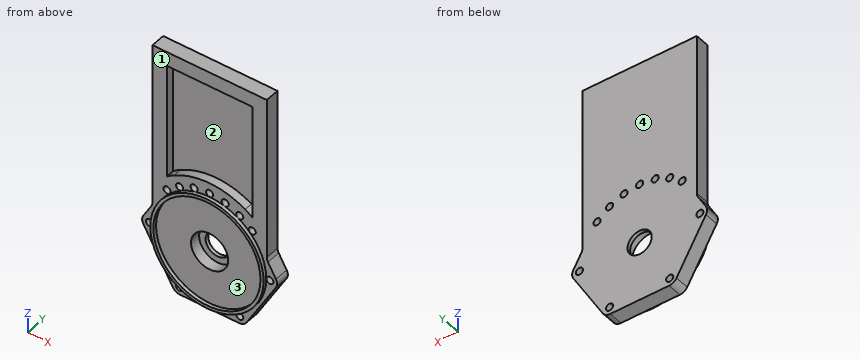
Autodesk Inventor part; units mm, degrees
ref_plane "YZ Plane" through (0, 0, 0) normal (1, 0, 0) x (0, 1, 0)
ref_plane "XZ Plane" through (0, 0, 0) normal (0, 1, 0) x (-1, 0, 0)
ref_plane "XY Plane" through (0, 0, 0) normal (0, 0, 1) x (1, 0, 0)
sketch "Sketch1" plane through (0, 0, 0) normal (0, 1, 0) x (-1, 0, 0)
  line L0 (83.678612, 197.794487) -> (-76.321388, 197.794487)
  line L1 (-76.321388, 197.794487) -> (-76.321388, -52.205513)
  line L2 (-76.321388, -52.205513) -> (83.678612, -52.205513)
  line L3 (83.678612, -52.205513) -> (83.678612, 197.794487)
  circle A0 centre (3.678612, -62.205513) radius 80
  line L4 (83.678612, -52.205513) -> (83.678612, -62.205513)
  line L5 (-76.321388, -52.205513) -> (-76.321388, -62.205513)
  circle A1 centre (3.678612, -62.205513) radius 26
  circle A2 centre (3.678612, -62.205513) radius 40
  point P0 (0, 0)
  point P1 (59.392898, -23.634084)
  point P2 (-75.693927, -52.205513)
  point P3 (83.051152, -52.205513)
  dimension "d0" = 250
  dimension "d1" = 160
  dimension "d2" = 160
  dimension "d3" = 10
  dimension "d4" = 52
  dimension "d5" = 80
extrude "Extrusion1" add sketch "Sketch1" along normal blind 20 contours L3 L2 A0 L1 L0 | L4 A0 L2 | L2 A0 L5 | A0 L2 A2 | L2 A2 A0 | A2 L2 A1 | L2 A1 A2
sketch "Sketch2" plane through (0, 20, 0) normal (0, 1, 0) x (1, 0, 0)
  circle A0 centre (-3.678612, 62.205513) radius 26
  circle A1 centre (-3.678612, 62.205513) radius 26
  circle A2 centre (-3.678612, 62.205513) radius 17
  point P0 (0, 0)
  dimension "d8" = 34
extrude "Extrusion2" add sketch "Sketch2" against normal blind 5
sketch "Sketch3" plane through (0, 0, 0) normal (0, -1, 0) x (1, 0, 0)
  circle A0 centre (-3.678612, -62.205513) radius 75
  circle A1 centre (-3.678612, -62.205513) radius 75
  line L0 (92.607102, -62.205513) -> (44.464245, -145.591387)
  line L1 (44.464245, -145.591387) -> (-51.821469, -145.591387)
  line L2 (-51.821469, -145.591387) -> (-99.964327, -62.205513)
  line L3 (-99.964327, -62.205513) -> (-51.821469, 21.180362)
  line L4 (-51.821469, 21.180362) -> (44.464245, 21.180362)
  line L5 (44.464245, 21.180362) -> (92.607102, -62.205513)
  line L6 (80.607102, -62.205513) -> (38.464245, -135.199083)
  line L7 (38.464245, -135.199083) -> (-45.821469, -135.199083)
  line L8 (-45.821469, -135.199083) -> (-87.964327, -62.205513)
  line L9 (-87.964327, -62.205513) -> (-45.821469, 10.788057)
  line L10 (-45.821469, 10.788057) -> (38.464245, 10.788057)
  line L11 (38.464245, 10.788057) -> (80.607102, -62.205513)
  circle A2 centre (80.607102, -62.205513) radius 5
  circle A3 centre (38.464245, 10.788057) radius 5
  circle A4 centre (-45.821469, 10.788057) radius 5
  circle A5 centre (-87.964327, -62.205513) radius 5
  circle A6 centre (-45.821469, -135.199083) radius 5
  circle A7 centre (38.464245, -135.199083) radius 5
  circle A8 centre (-3.678612, -62.205513) radius 26
  circle A9 centre (-3.678612, -62.205513) radius 0.853538
  point P0 (0, 0)
  point P1 (-59.392898, -100.776941)
  point P2 (-3.678612, -62.205513)
  dimension "d13" = 360
sketch "Sketch4" plane through (0, 0, 0) normal (0, -1, 0) x (1, 0, 0)
  circle A0 centre (-45.821469, -135.199083) radius 5
  line L0 (-45.821469, -135.199083) -> (-87.964327, -62.205513)
  line L1 (-51.821469, -145.591387) -> (-99.964327, -62.205513)
  circle A1 centre (-87.964327, -62.205513) radius 5
  circle A2 centre (-45.821469, 10.788057) radius 5
  line L2 (-87.964327, -62.205513) -> (-45.821469, 10.788057)
  line L3 (-99.964327, -62.205513) -> (-51.821469, 21.180362)
  line L4 (38.464245, -135.199083) -> (-45.821469, -135.199083)
  circle A3 centre (38.464245, -135.199083) radius 5
  line L5 (44.464245, -145.591387) -> (-51.821469, -145.591387)
  line L6 (80.607102, -62.205513) -> (38.464245, -135.199083)
  line L7 (92.607102, -62.205513) -> (44.464245, -145.591387)
  circle A4 centre (-3.678612, -62.205513) radius 75
  circle A5 centre (-3.678612, -62.205513) radius 75
  line L8 (-45.821469, 10.788057) -> (38.464245, 10.788057)
  line L9 (-51.821469, 21.180362) -> (44.464245, 21.180362)
  circle A6 centre (80.607102, -62.205513) radius 5
  circle A7 centre (38.464245, 10.788057) radius 5
  line L10 (38.464245, 10.788057) -> (80.607102, -62.205513)
  line L11 (44.464245, 21.180362) -> (92.607102, -62.205513)
  circle A8 centre (-3.678612, -62.205513) radius 26
  circle A9 centre (-3.678612, -62.205513) radius 17
  circle A10 centre (-3.678612, -62.205513) radius 2.321388
  point P0 (0, 0)
  point P1 (0, 0)
  point P2 (-59.392898, -100.776941)
  dimension "d18" = 360
extrude "Extrusion3" cut sketch "Sketch3" against normal blind 22 contours A2 L6 L11 | L11 L6 A2 | A3 L10 L11 | L11 L10 A3 | A7 L7 L6 | L6 L7 A7 | A4 L9 L10 | L10 L9 A4 | A6 L8 L7 | L7 L8 A6 | A5 L8 L9 | L9 L8 A5
extrude "Extrusion4" add sketch "Sketch4" against normal blind 20 contours A0 L0 A4 L4 | A4 L6 A3 L4 | L0 A1 L2 A4 | A4 L10 A6 L6 | L2 A2 L8 A4 | L8 A7 L10 A4 | L1 L3 L9 L11 L7 L5
sketch "Sketch5" plane through (0, 0, 0) normal (0, -1, 0) x (1, 0, 0)
  circle A0 centre (-3.678612, -62.205513) radius 17
  circle A1 centre (-3.678612, -62.205513) radius 79.285714
  circle A2 centre (80.607102, -62.205513) radius 5
  circle A3 centre (-3.678612, -62.205513) radius 75
  point P0 (0, 0)
  dimension "d21" = 150
extrude "Extrusion5" add sketch "Sketch5" along normal blind 5 contours A1
fillet "Fillet1" radius 12 6 edges at (-83.6786, 10, -33.9978) (-99.9643, 10, -62.2055) (-51.8215, 10, -145.5914) (44.4642, 10, -145.5914) (92.6071, 10, -62.2055) (76.3214, 10, -33.9978)
sketch "Sketch6" plane through (0, 0, 0) normal (0, -1, 0) x (1, 0, 0)
  arc A0 (89.143, -68.205513) -> (89.143, -56.205513) centre (78.750696, -62.205513) ccw
  line L0 (89.143, -56.205513) -> (77.929083, -36.782438)
  arc A1 (76.321388, -30.782438) -> (77.929083, -36.782438) centre (88.321388, -30.782438) ccw
  line L1 (76.321388, 197.794487) -> (76.321388, -30.782438)
  line L2 (-83.678612, 197.794487) -> (76.321388, 197.794487)
  line L3 (-83.678612, -30.782438) -> (-83.678612, 197.794487)
  arc A2 (-85.286307, -36.782438) -> (-83.678612, -30.782438) centre (-95.678612, -30.782438) ccw
  line L4 (-85.286307, -36.782438) -> (-96.500225, -56.205513)
  arc A3 (-96.500225, -56.205513) -> (-96.500225, -68.205513) centre (-86.10792, -62.205513) ccw
  line L5 (-96.500225, -68.205513) -> (-55.285571, -139.591387)
  arc A4 (-55.285571, -139.591387) -> (-44.893266, -145.591387) centre (-44.893266, -133.591387) ccw
  line L6 (-44.893266, -145.591387) -> (37.536042, -145.591387)
  arc A5 (37.536042, -145.591387) -> (47.928346, -139.591387) centre (37.536042, -133.591387) ccw
  line L7 (47.928346, -139.591387) -> (89.143, -68.205513)
  circle A6 centre (-87.964327, -62.205513) radius 5
  arc A7 (-43.321469, 6.45793) -> (-82.964327, -62.205513) centre (-3.678612, -62.205513) ccw
  circle A8 centre (-45.821469, 10.788057) radius 5
  arc A9 (35.964245, 6.45793) -> (-43.321469, 6.45793) centre (-3.678612, -62.205513) ccw
  circle A10 centre (38.464245, 10.788057) radius 5
  arc A11 (75.607102, -62.205513) -> (35.964245, 6.45793) centre (-3.678612, -62.205513) ccw
  circle A12 centre (80.607102, -62.205513) radius 5
  arc A13 (35.964245, -130.868956) -> (75.607102, -62.205513) centre (-3.678612, -62.205513) ccw
  circle A14 centre (38.464245, -135.199083) radius 5
  arc A15 (-43.321469, -130.868956) -> (35.964245, -130.868956) centre (-3.678612, -62.205513) ccw
  circle A16 centre (-45.821469, -135.199083) radius 5
  arc A17 (-82.964327, -62.205513) -> (-43.321469, -130.868956) centre (-3.678612, -62.205513) ccw
  arc A18 (56.321388, -30.782438) -> (60.608575, -46.782438) centre (88.321388, -30.782438) ccw
  line L8 (60.608575, -46.782438) -> (69.513091, -62.205513)
  line L9 (69.513091, -62.205513) -> (32.917239, -125.591387)
  line L10 (32.917239, -125.591387) -> (-40.274464, -125.591387)
  line L11 (-40.274464, -125.591387) -> (-76.870316, -62.205513)
  line L12 (-76.870316, -62.205513) -> (-67.965799, -46.782438)
  arc A19 (-67.965799, -46.782438) -> (-63.678612, -30.782438) centre (-95.678612, -30.782438) ccw
  line L13 (-63.678612, -30.782438) -> (-63.678612, 177.794487)
  line L14 (-63.678612, 177.794487) -> (56.321388, 177.794487)
  line L15 (56.321388, 177.794487) -> (56.321388, -30.782438)
  arc A20 (-53.321469, 23.778438) -> (-102.964327, -62.205513) centre (-3.678612, -62.205513) ccw
  arc A21 (-102.964327, -62.205513) -> (-53.321469, -148.189464) centre (-3.678612, -62.205513) ccw
  arc A22 (-53.321469, -148.189464) -> (45.964245, -148.189464) centre (-3.678612, -62.205513) ccw
  arc A23 (45.964245, -148.189464) -> (95.607102, -62.205513) centre (-3.678612, -62.205513) ccw
  arc A24 (95.607102, -62.205513) -> (45.964245, 23.778438) centre (-3.678612, -62.205513) ccw
  arc A25 (45.964245, 23.778438) -> (-53.321469, 23.778438) centre (-3.678612, -62.205513) ccw
  point P0 (0, 0)
  point P1 (-63.678612, 16.899816)
  point P2 (56.321388, 16.899816)
  dimension "d25" = 20
  dimension "d26" = 20
sketch "Sketch6 outline for Extrusion6" plane through (0, 0, 0) normal (0, -1, 0) x (1, 0, 0)
  line L0 (56.321388, 177.794487) -> (-63.678612, 177.794487)
  line L1 (56.321388, 16.899816) -> (56.321388, 177.794487)
  arc A0 (45.964245, 23.778438) -> (56.321388, 16.899816) centre (-3.678612, -62.205513) cw
  arc A1 (-53.321469, 23.778438) -> (45.964245, 23.778438) centre (-3.678612, -62.205513) cw
  arc A2 (-63.678612, 16.899816) -> (-53.321469, 23.778438) centre (-3.678612, -62.205513) cw
  line L2 (-63.678612, 177.794487) -> (-63.678612, 16.899816)
extrude "Extrusion6" cut sketch "Sketch6 outline for Extrusion6" against normal blind 12
sketch "Sketch7" plane through (0, 0, 0) normal (0, -1, 0) x (1, 0, 0)
  circle A0 centre (-3.678612, 22.080487) radius 5
  circle A1 centre (-3.678612, -62.205513) radius 17
  circle A2 centre (-25.493434, 19.208511) radius 5
  circle A3 centre (-45.821612, 10.788304) radius 5
  circle A4 centre (-63.277814, -2.606311) radius 5
  circle A5 centre (-76.672429, -20.062513) radius 5
  circle A6 centre (-85.092637, -40.390691) radius 5
  circle A7 centre (-87.964612, -62.205513) radius 5
  circle A8 centre (-85.092637, -84.020335) radius 5
  circle A9 centre (-76.672429, -104.348513) radius 5
  circle A10 centre (-63.277814, -121.804715) radius 5
  circle A11 centre (-45.821612, -135.19933) radius 5
  circle A12 centre (-25.493434, -143.619537) radius 5
  circle A13 centre (-3.678612, -146.491513) radius 5
  circle A14 centre (18.13621, -143.619537) radius 5
  circle A15 centre (38.464388, -135.19933) radius 5
  circle A16 centre (55.92059, -121.804715) radius 5
  circle A17 centre (69.315205, -104.348513) radius 5
  circle A18 centre (77.735412, -84.020335) radius 5
  circle A19 centre (80.607388, -62.205513) radius 5
  circle A20 centre (77.735412, -40.390691) radius 5
  circle A21 centre (69.315205, -20.062513) radius 5
  circle A22 centre (55.92059, -2.606311) radius 5
  circle A23 centre (38.464388, 10.788304) radius 5
  circle A24 centre (18.13621, 19.208511) radius 5
  point P0 (0, 0)
  dimension "d29" = 84.286
  dimension "d30" = 10
  dimension "d33" = 360
extrude "Extrusion7" cut sketch "Sketch7" against normal blind 39 contours A0 | A2 | A4 | A5 | A21 | A22 | A24
sketch "Sketch8" plane through (0, 20, 0) normal (0, 1, 0) x (1, 0, 0)
  circle A0 centre (69.315205, 20.062513) radius 5
  circle A1 centre (-76.672429, 20.062513) radius 5
  point P0 (0, 0)
extrude "Extrusion8" add sketch "Sketch8" against normal blind 20
properties part number "ZadKriska"
Here's how the part is built. I have some questions about the finished solid (model axes, mm). Face numbers are marked on the shaded views. A direction names the side the tool comes from. Round coordinates to 2 decimals unless told otherwise and drop trailing zeros. Order: outer loops, then holes, each group sorted by start corner. A loop starts at its lowest first (then second) coordinate and runs counter-clockwise, first axis right, second up. Notation, with made-up numbers: M 32,22 L 63,22 A33 cw 63,60 Z; hole C -29,48 d1. An arc over 180 degrees is marked long. Return JSON: item names as keys, results as strings. Group by question number.
1. If we section it at B-B on z = -50: List the corners of the cut face in (x, y) for me, then the cut area to 3 significant figures.
2. If we section it at A-A on z = 153: List the corners of the cut face in (x, y) for me.
3. On a 3-axis mill with a long thin cutter (end or side, diameter ignored), from which of +Z, -Z, +X, -X, +Y, -Y can I reach the whole of each face in a straight line? I mean the marked faces 3 and 4. Say none if no direction works.
4. Please list where these lines run through material, in increasing order: probe 1 along Z at (x, y) = (-4.5, 17.5); probe 2 along Z at (x, y) = (-4.5, -3.25); probe 3 along Z at (x, y) = (-50, 2).
5. If we section it at C-C on y = 4.75: State how many separate pieces and enclosed holes the cut face has, then the cut area to 3 significant figures.
6. If we section it at D-D on x = 28: List the corners of the cut face in (y, z) for me.
7. I'm going to push flat-ended pins straight in: pin 1 Ø8 at (x, z) = (80.61, -62.21) entering from -Y; pin 2 Ø11.5 at (x, z) = (-87.96, -62.21) entering from +Y; pin 3 Ø5 at (y, z) = (-0.5, 115.5) entering from +X; pin 4 Ø3 at (x, z) = (18.5, 63.5) entering from -Y. Where does each tip first touch, or does it pass through?
8. If we mould it in two halves opening along X, with no side actions, what happens to the marked faces 1 and 2? For each: pulls with the +X half, pulls with the -X half, needs draft (parallel to the pull), parting line crosses it, or undercut.
Reply:
{
 "1": {"outline": "M -92.92,0 L -82.02,0 L -82.02,-5 L -77.68,-5 L -77.68,0 L -26.64,0 L -26.64,15 L -15.51,15 L -15.51,20 L -92.92,20 Z; M 8.15,15 L 19.28,15 L 19.28,0 L 70.32,0 L 70.32,-5 L 74.66,-5 L 74.66,0 L 85.56,0 L 85.56,20 L 8.15,20 Z", "area": "2,810 mm^2"},
 "2": {"outline": "M -83.68,0 L -63.68,0 L -63.68,12 L 56.32,12 L 56.32,0 L 76.32,0 L 76.32,20 L -83.68,20 Z"},
 "3": {"face 3": "-Y", "face 4": "+Z, -Z, +X, -X, +Y"},
 "4": {"probe 1": "-145.59 to -79.19, -45.23 to 17.15, 27.01 to 197.79", "probe 2": "-141.49 to -137.2, 12.79 to 17.08", "probe 3": "-144.45 to -137.94, -132.45 to 8.04, 13.53 to 25.61, 177.79 to 197.79"},
 "5": {"separate pieces": "1", "enclosed holes": "13", "area": "33,400 mm^2"},
 "6": {"outline": "M -5,-134.89 L 0,-134.89 L 0,-145.59 L 20,-145.59 L 20,197.79 L 0,197.79 L 0,177.79 L 12,177.79 L 12,31.89 L 0,31.89 L 0,10.48 L -5,10.48 L -5,5.78 L 0,5.78 L 0,-130.19 L -5,-130.19 Z"},
 "7": {"pin 1": "through", "pin 2": "y = 20", "pin 3": "x = 76.32", "pin 4": "y = 12"},
 "8": {"face 1": "needs draft", "face 2": "undercut"}
}
